Source: CAD feature listing. Evaluate the final solid. Frame: model axes, mm. A direction names the side the tool comes from. Coordinates: 2 decimals unless noted, no trailing zeros. Order: outer loops, then holes, each group sorted by start corner. A loop starts at its lowest first (then second) coordinate and runs counter-clockwise, first axis right, second up.
```python
from build123d import *

# Parameters (mm, degrees)
SKETCH1_W           = 36.024962638
SKETCH1_H           = 38.826904176
SKETCH1_R           = 1.397
SKETCH1_R_2         = 2.5527
BOSS_EXTRUDE1_DEPTH = 3.175


with BuildPart() as part:
    # Sketch1 → Boss-Extrude1 (new body)
    with BuildSketch(Plane.XY):
        with Locations((34.711147671, -14.342506761)):
            Rectangle(SKETCH1_W, SKETCH1_H)
        with Locations((45.918913825, -2.000621413)):
            Circle(SKETCH1_R, mode=Mode.SUBTRACT)
        with Locations((23.503381517, -2.000621413)):
            Circle(SKETCH1_R, mode=Mode.SUBTRACT)
        with Locations((23.503381517, -26.684392109)):
            Circle(SKETCH1_R, mode=Mode.SUBTRACT)
        with Locations((45.918913825, -26.684392109)):
            Circle(SKETCH1_R, mode=Mode.SUBTRACT)
        with Locations((34.711147671, -6.937375552)):
            Circle(SKETCH1_R_2, mode=Mode.SUBTRACT)
        Polygon((40.210408985, -19.079122219), (37.460778328, -14.316622219), (31.961517014, -14.316622219), (29.211886357, -19.079122219), (31.961517014, -23.841622219), (37.460778328, -23.841622219), align=None, mode=Mode.SUBTRACT)
    extrude(amount=BOSS_EXTRUDE1_DEPTH)


solid = part.part
```
1. Section query D-D on x = 36.5. Return loops of the section in (y, z) (3 decimals), plus the area to 3 significant figures.
Findings:
outline: (-33.756, 0) - (-23.842, 0) - (-23.842, 3.175) - (-33.756, 3.175) - close; (-14.317, 0) - (-8.758, 0) - (-8.758, 3.175) - (-14.317, 3.175) - close; (-5.116, 0) - (5.071, 0) - (5.071, 3.175) - (-5.116, 3.175) - close
area: 81.5 mm2
2. Section query A-A on y = -18.5. Return loops of the section in (x, z) (3 decimals).
Findings:
outline: (16.699, 0) - (29.546, 0) - (29.546, 3.175) - (16.699, 3.175) - close; (39.876, 0) - (52.724, 0) - (52.724, 3.175) - (39.876, 3.175) - close
3. Section query C-C on z = 1.95. Return loops of the section in (x, y), plus the area to 3 significant figures.
Findings:
outline: (16.7, -33.76) - (52.72, -33.76) - (52.72, 5.07) - (16.7, 5.07) - close; hole circle Ø2.79 at (23.5, -26.68); hole circle Ø2.79 at (23.5, -2); hole (29.21, -19.08) - (31.96, -23.84) - (37.46, -23.84) - (40.21, -19.08) - (37.46, -14.32) - (31.96, -14.32) - close; hole circle Ø5.11 at (34.71, -6.94); hole circle Ø2.79 at (45.92, -26.68); hole circle Ø2.79 at (45.92, -2)
area: 1,280 mm2
4. Access query for faces 1 (the face through (30.61, -16.66, 1.57)), 2 (the face through (34, -14, 0)). Directions: +Z, -Z, +X, -X, +Y, -Y. A direction counts if a zero-diameter tool reaches every point of the face in a straight line with its end or side. Return the directions, or none.
Findings:
face 1: +Z, -Z
face 2: -Z, +X, -X, +Y, -Y
5. Pin query (flat end, axial travel): P1, Ø4, axis at x = 47, y = -2.5, coming from the -Z side; P2, Ø2.5, axis at x = 45.92, y = -2, coming from the -Z side. Return the tip coordinate at first contact, or that it passes through.
Findings:
P1: stops at z = 0
P2: passes through
6. Section query B-B on x = 30. Return loops of the section in (y, z) (3 decimals), plus the area to 3 significant figures.
Findings:
outline: (-33.756, 0) - (-20.444, 0) - (-20.444, 3.175) - (-33.756, 3.175) - close; (-17.714, 0) - (5.071, 0) - (5.071, 3.175) - (-17.714, 3.175) - close
area: 115 mm2
7. Ray query, line 1 (Y direction, x = 46, z = 2.85); line 2 (Y direction, x = 34, z = 1.25); line 3 (X direction, y = -2.5, z = 0.2). Return the intervals inside material, ascending.
Findings:
line 1: y = -33.76 to -28.08, -25.29 to -3.4, -0.61 to 5.07
line 2: y = -33.76 to -23.84, -14.32 to -9.39, -4.49 to 5.07
line 3: x = 16.7 to 22.2, 24.81 to 44.61, 47.22 to 52.72
8. Draft query along Y for faces 3 (the face through (16.699, -15, 2)), 4 (the face through (34, -33.756, 2)), 5 (the face through (35, -23.842, 2)). Return one class per face: released by +Y, released by -Y, zero draft, split by the parting line, or undercut.
Findings:
face 3: zero draft
face 4: released by -Y
face 5: undercut
